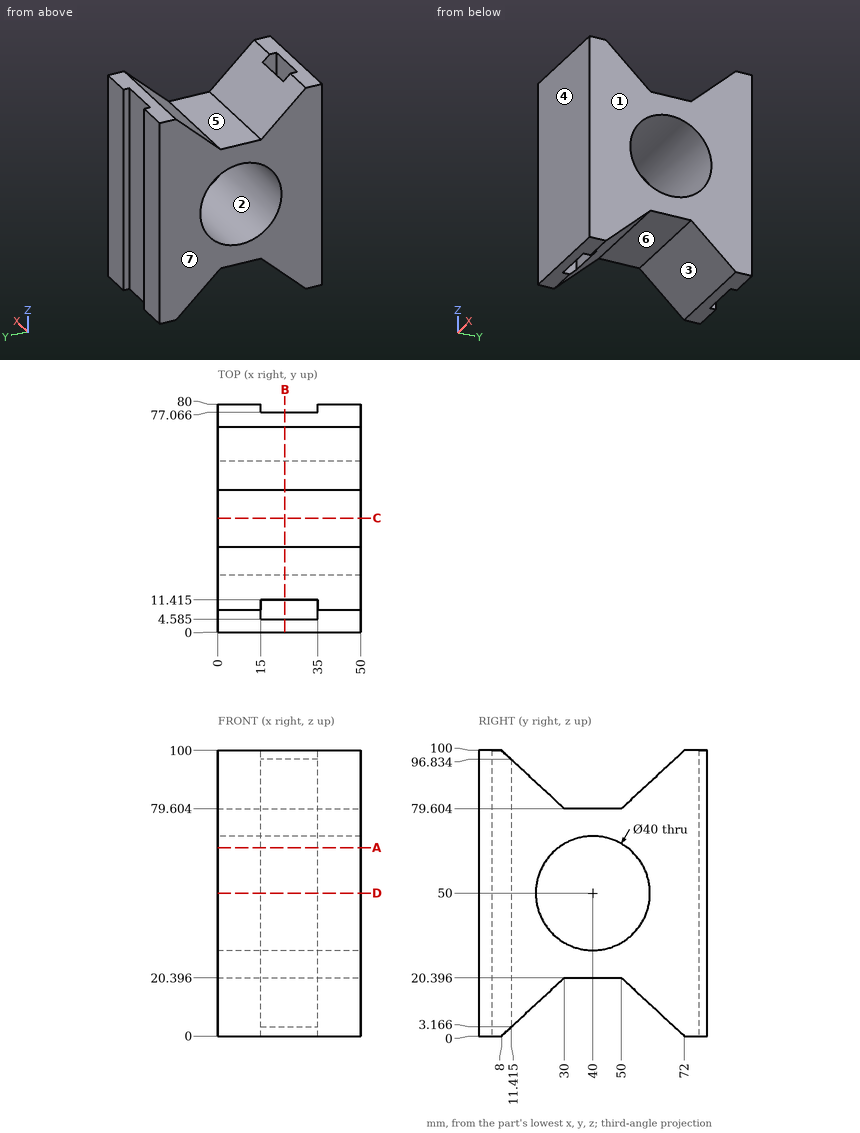
The drawing under review shows one solid part. Ordinate dimensions are in mm from its lowest x, y, z. A direction names the side the tool comes from. Coordinates: 2 decimals unless noted, no trailing zeros. Write each loop counter-clockwise with the first axis right and the second up, starting at its lowest first coordinate (ties: lowest second). Pieces come first, ordered by that corner, then holes. Notation, with made-up numbers: (68, 65) -> (105, 65) arc R8 cw to (105, 73) -> close; hole circle Ø5 at (71, -14.75). An arc over 180 degrees is marked (long way). One line per item, written item: value. Start each with the question number.
Q1. Add section D-D, the plane z = 50. Give the boundary of the cut face in (x, y) (1 decimal), then the cut area to 3 significant figures.
Q2. Add section A-A, the plane z = 66. Give the boundary of the cut face in (x, y) (1 decimal), then the cut area to 3 significant figures.
Q3. To check wall thickness, follow probe 1 along Y at (x, z) = (26, 50) (1 decimal); probe 2 along Y at (x, z) = (21, 81) (1 decimal); probe 3 along Y at (x, z) = (12, 50). State the ranges of each line that lie inside material, in increasing order.
Q4. Clearance check with flat-ended pins moving along their axes: P1, Ø4, axis at x = 18, y = 43, coming from the +Z side; P2, Ø6, axis at x = 20.5, z = 74.5, coming from the +Y side; P3, Ø22, axis at x = 21.5, y = 38.5, coming from the +Z side; P4, Ø3, axis at y = 55, z = 39.5, coming from the +X side. State where each tip first meets the part, or that it passes through.
Q5. The part is to be moulded in two halves that separate along Y. For the marked faces 1, 2, 3 and 4, say which applies: +Y half, -Y half, draft (parallel to the pull), parting line (faces both ways), or undercut.
Q6. Add section B-B, the plane x = 23.5. Give the boundary of the cut face in (y, z) (1 decimal), then the cut area to 3 significant figures.
Q7. Add section C-C, the plane y = 40. Give the boundary of the cut face in (x, z).
Q8. For the marked faces 5, 6 and 7, list the 3-axis set-ups (+Z, -Z, +X, -X, +Y, -Y) from which the entire face can be reached by the end or side of a thin tool; tool diameter is ignored.
Response:
1. outline: (0, 0) -> (50, 0) -> (50, 20) -> (0, 20) -> close; (0, 60) -> (50, 60) -> (50, 80) -> (35, 80) -> (35, 77.1) -> (15, 77.1) -> (15, 80) -> (0, 80) -> close; hole (15, 4.6) -> (35, 4.6) -> (35, 11.4) -> (15, 11.4) -> close
1. area: 1,800 mm²
2. outline: (0, 0) -> (50, 0) -> (50, 28) -> (0, 28) -> close; (0, 52) -> (50, 52) -> (50, 80) -> (35, 80) -> (35, 77.1) -> (15, 77.1) -> (15, 80) -> (0, 80) -> close; hole (15, 4.6) -> (35, 4.6) -> (35, 11.4) -> (15, 11.4) -> close
2. area: 2,600 mm²
3. probe 1: 0 to 4.6, 11.4 to 20, 60 to 77.1
3. probe 2: 0 to 4.6, 11.4 to 28.5, 51.5 to 77.1
3. probe 3: 0 to 20, 60 to 80
4. P1: z = 79.6
4. P2: y = 77.07
4. P3: z = 81.92
4. P4: through
5. face 1: draft
5. face 2: undercut
5. face 3: undercut
5. face 4: -Y half
6. outline: (0, 0) -> (4.6, 0) -> (4.6, 100) -> (0, 100) -> close; (11.4, 3.2) -> (30, 20.4) -> (50, 20.4) -> (72, 0) -> (77.1, 0) -> (77.1, 100) -> (72, 100) -> (50, 79.6) -> (30, 79.6) -> (11.4, 96.8) -> close; hole circle Ø40 at (40, 50)
6. area: 4,060 mm²
7. outline: (0, 20.4) -> (50, 20.4) -> (50, 30) -> (0, 30) -> close; (0, 70) -> (50, 70) -> (50, 79.6) -> (0, 79.6) -> close
8. face 5: +Z, +X, -X
8. face 6: -Z, +X, -X
8. face 7: +Z, -Z, -X, +Y, -Y
